from build123d import *

# Parameters (mm, degrees)
F0_W      = 120
F0_H      = 28
F1_DEPTH  = 8.6
F3_DEPTH  = 8.601
F2_R      = 40.1
F2_R_2    = 29.1
F4_DEPTH  = 8.6
F6_R      = 4.1
F7_DEPTH  = 8.601
F9_DEPTH  = 22.2
F11_DEPTH = 22.2
F12_R     = 36.3
F12_R_2   = 29.1
F13_DEPTH = 6.6


with BuildPart() as f1:
    # F0 (on Front) → F1 (new body)
    with BuildSketch(Plane.XZ):
        Rectangle(F0_W, F0_H)
    extrude(amount=F1_DEPTH)

    # F2 (on face) → F3 (cut, through all)
    with BuildSketch(Plane.XZ.offset(8.6)):
        with BuildLine():
            Line((-25.5109780291, 14), (25.5109780291, 14))
            ThreePointArc((25.5109780291, 14), (0, 29.1), (-25.5109780291, 14))
        make_face()
        with BuildLine():
            ThreePointArc((29.1, 0), (28.1884680379, 7.2263593653), (25.5109780291, 14))
            Line((25.5109780291, 14), (-25.5109780291, 14))
            ThreePointArc((-25.5109780291, 14), (-29.1, 0), (-25.5109780291, -14))
            Line((-25.5109780291, -14), (25.5109780291, -14))
            ThreePointArc((25.5109780291, -14), (28.1884680379, -7.2263593653), (29.1, 0))
        make_face()
        with BuildLine():
            ThreePointArc((-25.5109780291, -14), (0, -29.1), (25.5109780291, -14))
            Line((25.5109780291, -14), (-25.5109780291, -14))
        make_face()
    extrude(amount=-F3_DEPTH, mode=Mode.SUBTRACT)


with BuildPart() as f4:
    # F2 (on face) → F4 (new body)
    with BuildSketch(Plane.XZ.offset(8.6)):
        Circle(F2_R)
        Circle(F2_R_2, mode=Mode.SUBTRACT)
    extrude(amount=-F4_DEPTH)


with BuildPart() as f1_1:
    add(f1.part)

    # F5: union F4
    add(f4.part)

    # F6 (on face) → F7 (cut, through all)
    with BuildSketch(Plane.XZ.offset(8.6)):
        with Locations((-49, 0)):
            Circle(F6_R)
        with Locations((49, 0)):
            Circle(F6_R)
    extrude(amount=-F7_DEPTH, mode=Mode.SUBTRACT)

    # F8 (on face) → F9 (cut)
    with BuildSketch(Plane.YZ.offset(60)):
        with BuildLine():
            ThreePointArc((-8.6, 11.0471715837), (-4.5464050539, 13.2412311016), (0, 14))
            Line((0, 14), (-8.6, 14))
            Line((-8.6, 14), (-8.6, 11.0471715837))
        make_face()
        with BuildLine():
            Line((-8.6, -14), (0, -14))
            ThreePointArc((0, -14), (-4.5464050539, -13.2412311016), (-8.6, -11.0471715837))
            Line((-8.6, -11.0471715837), (-8.6, -14))
        make_face()
    extrude(amount=-F9_DEPTH, mode=Mode.SUBTRACT)

    # F10 (on face) → F11 (cut)
    with BuildSketch(Plane(origin=(-60, 0, 0), x_dir=(0, -1, 0), z_dir=(-1, 0, 0))):
        with BuildLine():
            Line((8.6, 14), (0, 14))
            ThreePointArc((0, 14), (4.5464050539, 13.2412311016), (8.6, 11.0471715837))
            Line((8.6, 11.0471715837), (8.6, 14))
        make_face()
        with BuildLine():
            ThreePointArc((8.6, -11.0471715837), (4.5464050539, -13.2412311016), (0, -14))
            Line((0, -14), (8.6, -14))
            Line((8.6, -14), (8.6, -11.0471715837))
        make_face()
    extrude(amount=-F11_DEPTH, mode=Mode.SUBTRACT)

    # F12 (on face) → F13 (cut)
    with BuildSketch(Plane(origin=(0, 0, 0), x_dir=(-1, 0, 0), z_dir=(0, 1, 0))):
        Circle(F12_R)
        Circle(F12_R_2, mode=Mode.SUBTRACT)
    extrude(amount=-F13_DEPTH, mode=Mode.SUBTRACT)


solid = f1_1.part
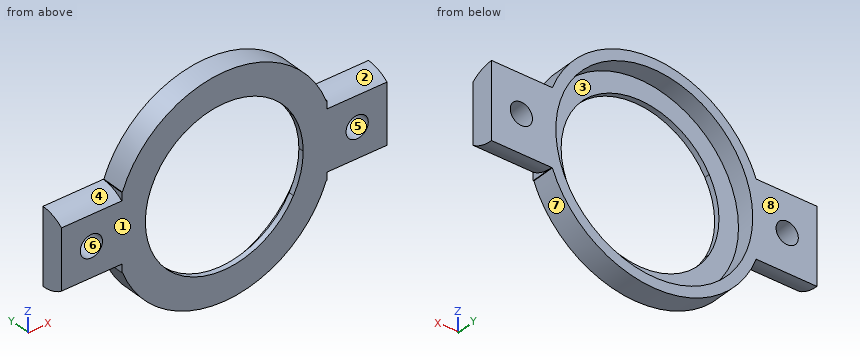
Can you work these out from the model? Positions are in its coordinate system, mm. Face numbers are marked on the shaded views. A direction names the side the tool comes from. Give positions to 0.01 mm unless a question says otherwise; leave off trailing zeros. Order: outer loops, then holes, each group sorted by start corner. A loop starts at its lowest first (then second) coordinate and runs counter-clockwise, first axis right, second up. Notation, with made-up numbers: M -21,21.25 L -17,21.25 A29 ccw -17,55.25 Z; hole C -1.75,4 d10. An arc over 180 degrees is marked long. One line per question, with ' | ' between items.
Item 1: Please list where these lines run through material, in increasing order: L1, parallel to Z at x = 0, y = -3.75; L2, parallel to X at y = -7.5, z = -2.5; L3, parallel to X at y = -6, z = 11.5.
Answer block:
L1: z = -40.1 to -36.3, 36.3 to 40.1 | L2: x = -60 to -52.25, -45.75 to -28.99, 28.99 to 45.75, 52.25 to 60 | L3: x = -60 to -34.43, 34.43 to 60
Item 2: For the marked faces 1, 2, 3 and 4, which set-ups out of +Z, -Z, +X, -X, +Y, -Y let a thin tool reach every point of the face, with its end or its side?
Answer block:
face 1: +Z, -Z, +X, -X, -Y | face 2: +Z, +X, -Y | face 3: +Y | face 4: +Z, -X, -Y
Item 3: Suppose I cut it at B-B, the plane z = -22. Write out the boundary of the cut face in (x, y), then the cut area to 3 significant figures.
Answer block:
outline: M -33.53,-8.6 L -19.05,-8.6 L -19.05,-6.6 L -28.87,-6.6 L -28.87,0 L -33.53,0 Z; M 19.05,-8.6 L 33.53,-8.6 L 33.53,0 L 28.87,0 L 28.87,-6.6 L 19.05,-6.6 Z | area: 119 mm2
Item 4: Suppose I cut it at D-D, the plane y = -3.25. Write out the boundary of the cut face in (x, z), then the cut area to 3 significant figures.
Answer block:
outline: M -60,-13.62 L -37.8,-13.62 L -37.8,-14 L -37.58,-14 A40.1 ccw 37.58,-14 L 37.8,-14 L 37.8,-13.62 L 60,-13.62 L 60,13.62 L 37.8,13.62 L 37.8,14 L 37.58,14 A40.1 ccw -37.58,14 L -37.8,14 L -37.8,13.62 L -60,13.62 Z; hole C -49,0 d8.2; hole C 0,0 d72.6; hole C 49,0 d8.2 | area: 1,930 mm2
Item 5: I'm going to push flat-ended pins straight in: pin 1 Ø2 at (x, y) = (-19.5, -2.5) entering from -Z; pin 2 Ø1 at (x, y) = (6, -6) entering from +Z; pin 3 Ø22 at (x, z) = (16, 13.5) entering from +Y. Where does each tip first touch, or does it pass through?
Answer block:
pin 1: stops at z = -35.58 | pin 2: stops at z = 39.72 | pin 3: stops at y = -6.6
Item 6: Suppose I cut it at A-A, the plane x = 49. Write out the boundary of the cut face in (y, z), then the cut area to 3 significant figures.
Answer block:
outline: M -8.6,-11.05 A14 ccw 0,-14 L 0,-4.1 L -8.6,-4.1 Z; M -8.6,4.1 L 0,4.1 L 0,14 A14 ccw -8.6,11.05 Z | area: 154 mm2
Item 7: We'd pull the mould along X, two halves only. Please class the marked faces 5, 6, 7 and 8: released by +X, released by -X, zero draft, split by the parting line, or undercut.
Answer block:
face 5: undercut | face 6: undercut | face 7: split by the parting line | face 8: zero draft
Item 8: Suppose I cut it at C-C, the plane x = 0. Write out the boundary of the cut face in (y, z).
Answer block:
outline: M -8.6,-40.1 L 0,-40.1 L 0,-36.3 L -6.6,-36.3 L -6.6,-29.1 L -8.6,-29.1 Z; M -8.6,29.1 L -6.6,29.1 L -6.6,36.3 L 0,36.3 L 0,40.1 L -8.6,40.1 Z
